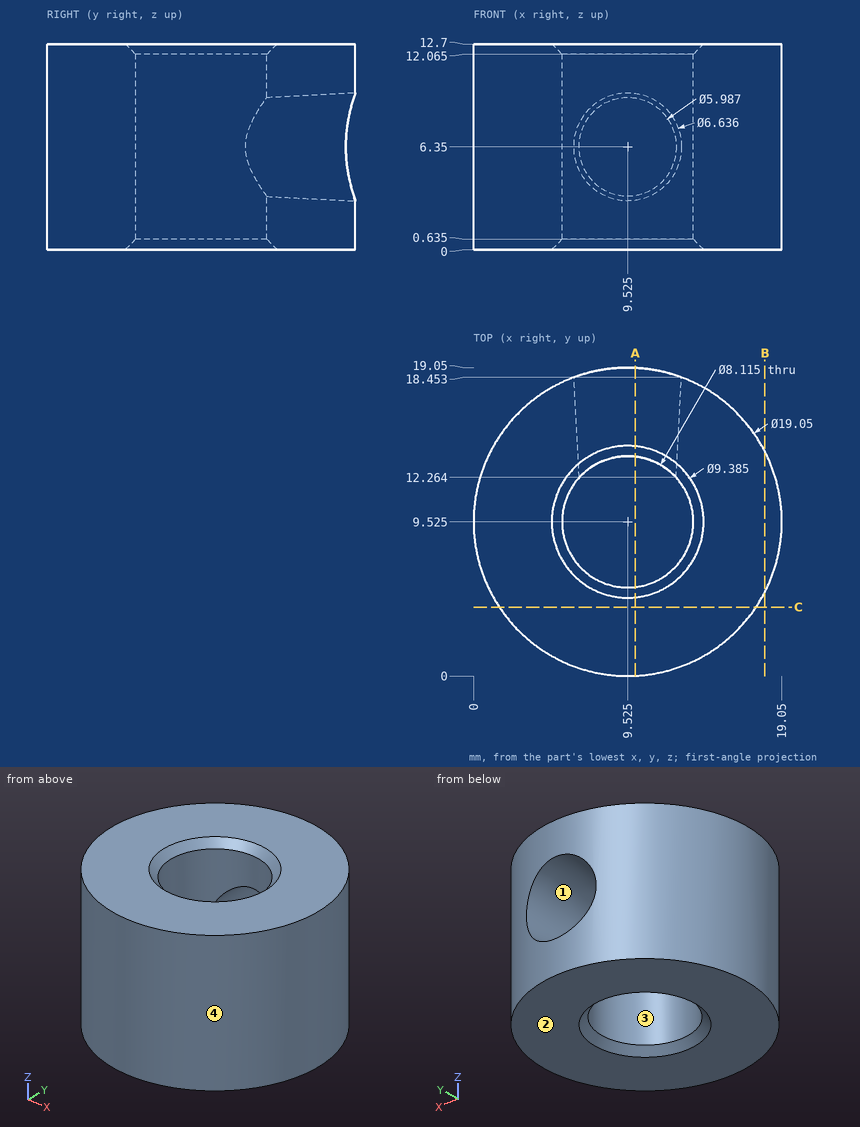
Could you check a few things on this drawing? It's one solid part, dimensions in mm from its lowest x, y, z. Give positions to 0.01 mm unless a question says otherwise; leave off trailing zeros. Order: outer loops, then holes, each group sorted by start corner. A loop starts at its lowest first (then second) coordinate and runs counter-clockwise, first axis right, second up. Notation, with made-up numbers: (38, 84.5) -> (74, 84.5) arc R21 ccw to (74, 120.5) -> close; hole circle Ø9 at (28, 22). An arc over 180 degrees is marked (long way). Use CSV: the item, a comma, the result in double quotes. Start each with the question number.
Item 1: If I drill on probe 1 along Z at (x, y) = (10, 15.5); probe 2 along X at (y, z) = (6.5, 9.5) (1 decimal); probe 3 along Y at (x, z) = (13.25, 11.5) (1 decimal), over which ranges is the centre line in solid material (lowest first)? Write a range as [from, to].
Item 2: I'm going to push flat-ended pins straight in: P1, Ø1.5, axis at x = 6, z = 9.5, coming from the -Y side; P2, Ø3, axis at y = 12.5, z = 9.5, coming from the -X side (1 decimal); P3, Ø1.5, axis at y = 12.5, z = 6, coming from the -X side. Where does each tip first touch, or does it pass through?
Item 3: Suppose I cut it at B-B (x = 18). List the corners of the cut face in (y, z) for me, and give its area (3 significant figures).
Item 4: Thinking about a two-plate mould opening in X: for the marked faces 1, 2, 3 and 4, which applies, pulls with the +X half, pulls with the -X half, needs draft (parallel to the pull), parting line crosses it, or undercut?
Item 5: Suppose I cut it at C-C (y = 4.25). List the corners of the cut face in (x, z) for me.
Item 6: Suppose I cut it at A-A (x = 10). Give the number of separate pieces and of enclosed holes in the cut face, and give its area (3 significant figures).
Answer block:
1,probe 1,"z = [0, 3.22], [9.48, 12.7]"
1,probe 2,"x = [0.5, 6.8], [12.2, 18.6]"
1,probe 3,"y = [0.8, 7.9], [11.1, 18.3]"
2,P1,"stops at y = 0.41"
2,P2,"stops at x = 0.1"
2,P3,"stops at x = 0.26"
3,outline,"(5.18, 0) -> (13.87, 0) -> (13.87, 12.7) -> (5.18, 12.7) -> close"
3,area,"110 mm^2"
4,face 1,"undercut"
4,face 2,"needs draft"
4,face 3,"undercut"
4,face 4,"parting line crosses it"
5,outline,"(1.59, 0) -> (17.46, 0) -> (17.46, 12.7) -> (1.59, 12.7) -> close"
6,separate pieces,"3"
6,enclosed holes,"0"
6,area,"104 mm^2"
